from build123d import *

# Parameters (mm, degrees)
BOSS_EXTRUDE1_DEPTH = 1700
SKETCH3_R           = 7
CUT_EXTRUDE1_DEPTH  = 10
SKETCH4_R           = 9
CUT_EXTRUDE2_DEPTH  = 20
LPATTERN1_COUNT     = 3
LPATTERN1_PITCH     = 805
SKETCH5_R           = 40
CUT_EXTRUDE3_DEPTH  = 30
LPATTERN2_COUNT     = 4
LPATTERN2_PITCH     = 366


with BuildPart() as part:
    # Sketch1 → Boss-Extrude1 (new body)
    with BuildSketch(Plane(origin=(0, 0, 0), x_dir=(0, 0, -1), z_dir=(1, 0, 0))):
        with BuildLine():
            Line((-86.622073579, 113.879598662), (-186.622073579, 113.879598662))
            Line((-186.622073579, 113.879598662), (-186.622073579, -186.120401338))
            Line((-186.622073579, -186.120401338), (-86.622073579, -186.120401338))
            Line((-86.622073579, -186.120401338), (-86.622073579, -180.120401338))
            ThreePointArc((-86.622073579, -180.120401338), (-89.551005767, -173.049333526), (-96.622073579, -170.120401338))
            Line((-96.622073579, -170.120401338), (-166.622073579, -170.120401338))
            ThreePointArc((-166.622073579, -170.120401338), (-173.69314139, -167.19146915), (-176.622073579, -160.120401338))
            Line((-176.622073579, -160.120401338), (-176.622073579, 87.879598662))
            ThreePointArc((-176.622073579, 87.879598662), (-173.69314139, 94.950666474), (-166.622073579, 97.879598662))
            Line((-166.622073579, 97.879598662), (-96.622073579, 97.879598662))
            ThreePointArc((-96.622073579, 97.879598662), (-89.551005767, 100.80853085), (-86.622073579, 107.879598662))
            Line((-86.622073579, 107.879598662), (-86.622073579, 113.879598662))
        make_face()
    extrude(amount=BOSS_EXTRUDE1_DEPTH)

    # Sketch3 → Cut-Extrude1 (cut)
    with BuildSketch(Plane.XY.offset(186.622073579)):
        with Locations((1655, 38.879598662)):
            Circle(SKETCH3_R)
        with Locations((1655, -36.120401338)):
            Circle(SKETCH3_R)
        with Locations((1655, -111.120401338)):
            Circle(SKETCH3_R)
    cut_extrude1 = extrude(amount=-CUT_EXTRUDE1_DEPTH, mode=Mode.SUBTRACT)

    # Mirror1: Cut-Extrude1 across plane
    add(cut_extrude1.mirror(Plane(origin=(850, 0, 0), x_dir=(0, 0, 1), z_dir=(1, 0, 0))), mode=Mode.SUBTRACT)

    # Sketch4 → Cut-Extrude2 (cut)
    with BuildSketch(Plane(origin=(0, 113.879598662, 0), x_dir=(1, 0, 0), z_dir=(0, 1, 0))):
        with Locations(Location((45, -131.622073579, 0), (0, 0, 270))):
            Circle(SKETCH4_R)
    cut_extrude2 = extrude(amount=-CUT_EXTRUDE2_DEPTH, mode=Mode.SUBTRACT)

    # LPattern1: Cut-Extrude2 ×3
    with Locations(*[(i * LPATTERN1_PITCH, 0, 0) for i in range(1, LPATTERN1_COUNT)]):
        add(cut_extrude2, mode=Mode.SUBTRACT)

    # Sketch5 → Cut-Extrude3 (cut)
    with BuildSketch(Plane(origin=(0, 0, 176.622073579), x_dir=(-1, 0, 0), z_dir=(0, 0, -1))):
        with Locations(Location((-1399, -36.120401338, 0), (0, 0, 90))):
            Circle(SKETCH5_R)
    cut_extrude3 = extrude(amount=-CUT_EXTRUDE3_DEPTH, mode=Mode.SUBTRACT)

    # LPattern2: Cut-Extrude3 ×4
    with Locations(*[(-i * LPATTERN2_PITCH, 0, 0) for i in range(1, LPATTERN2_COUNT)]):
        add(cut_extrude3, mode=Mode.SUBTRACT)


solid = part.part
Work out the finished part from the listing and answer in its coordinate system (mm). A direction names the side the tool comes from. Coordinates: 2 decimals unless noted, no trailing zeros. Loops run counter-clockwise (first coordinate to the right, second up) from the corner with the lowest first, then second, coordinate; pieces in that order, holes last. Notation, with made-up numbers: (15, 77.25) -> (63, 77.25) arc R17 ccw to (63, 93.25) -> close; hole circle Ø2 at (47, -9.5). An arc over 180 degrees is marked (long way). Write each question's results on one line, items separated by ' | '. Start each with the question number.
1) For faces 1 (the flat face through (1700, -13, 178)), 2 (the flat face through (838, -170.12, 131)), determine the directions among +Z, -Z, +X, -X, +Y, -Y from which every point of the face is accessible in a straight line to the end or side of a thin tool.
2) Find section A-A on x = 1399. Determine the outline of the cut face in (y, z), then the cut area to 3 significant figures.
3) Flat-ended cylindrical pins translate along their axes: P1, Ø5, axis at x = 1244, y = 57, coming from the -Z side; P2, Ø12.5, axis at x = 1655, y = -111.12, coming from the +Z side; P3, Ø11, axis at x = 45, z = 131.62, coming from the +Y side. Find the tip coordinate at first contact, or state that the pin passes through.
4) Consider line 1 along Y through (x, z) = (1655, 184); line 2 along Y through (x, z) = (1540, 119); line 3 along Z through (x, y) = (105, -161). Determine where each line is inside the solid, lowest interval first.
5) The mould has two halves that part along X. Classify faces 3 (the cylindrical face through (340.66, -41.33, 181.55)), 4 (the cylindrical face through (997.513, -17.663, 181.552)), 5 (the flat face through (838, 97.88, 132)), 6 (the flat face through (0, -13, 178)): pulls with the +X half, pulls with the -X half, needs draft (parallel to the pull), parting line crosses it, or undercut.
6) Find section B-B on x = 1220.5. Determine the outline of the cut face in (y, z).
Response values:
1) face 1: +Z, -Z, +X, +Y, -Y | face 2: -Z, +X, -X
2) outline: (-186.12, 86.62) -> (-180.12, 86.62) arc R10 ccw to (-170.12, 96.62) -> (-170.12, 166.62) arc R10 cw to (-160.12, 176.62) -> (-76.12, 176.62) -> (-76.12, 186.62) -> (-186.12, 186.62) -> close; (3.88, 176.62) -> (87.88, 176.62) arc R10 cw to (97.88, 166.62) -> (97.88, 96.62) arc R10 ccw to (107.88, 86.62) -> (113.88, 86.62) -> (113.88, 186.62) -> (3.88, 186.62) -> close | area: 5,080 mm^2
3) P1: stops at z = 176.62 | P2: passes through | P3: stops at y = -170.12
4) line 1: y = -186.12 to -118.12, -104.12 to -43.12, -29.12 to 31.88, 45.88 to 113.88 | line 2: y = -186.12 to -170.12, 97.88 to 113.88 | line 3: z = 176.58 to 186.62
5) face 3: undercut | face 4: undercut | face 5: needs draft | face 6: pulls with the -X half
6) outline: (-186.12, 86.62) -> (-180.12, 86.62) arc R10 ccw to (-170.12, 96.62) -> (-170.12, 166.62) arc R10 cw to (-160.12, 176.62) -> (87.88, 176.62) arc R10 cw to (97.88, 166.62) -> (97.88, 96.62) arc R10 ccw to (107.88, 86.62) -> (113.88, 86.62) -> (113.88, 186.62) -> (-186.12, 186.62) -> close
